Design review of the part shown in the three views and the two pictorial views. Dimensions are in mm from the part's minimum x, y and z. A direction names the side the tool comes from. Give positions to 0.01 mm unless a question says otherwise; leave off trailing zeros. Write each loop counter-clockwise with the first axis right and the second up, starting at its lowest first coordinate (ties: lowest second). Pieces come first, ordered by that corner, then holes.
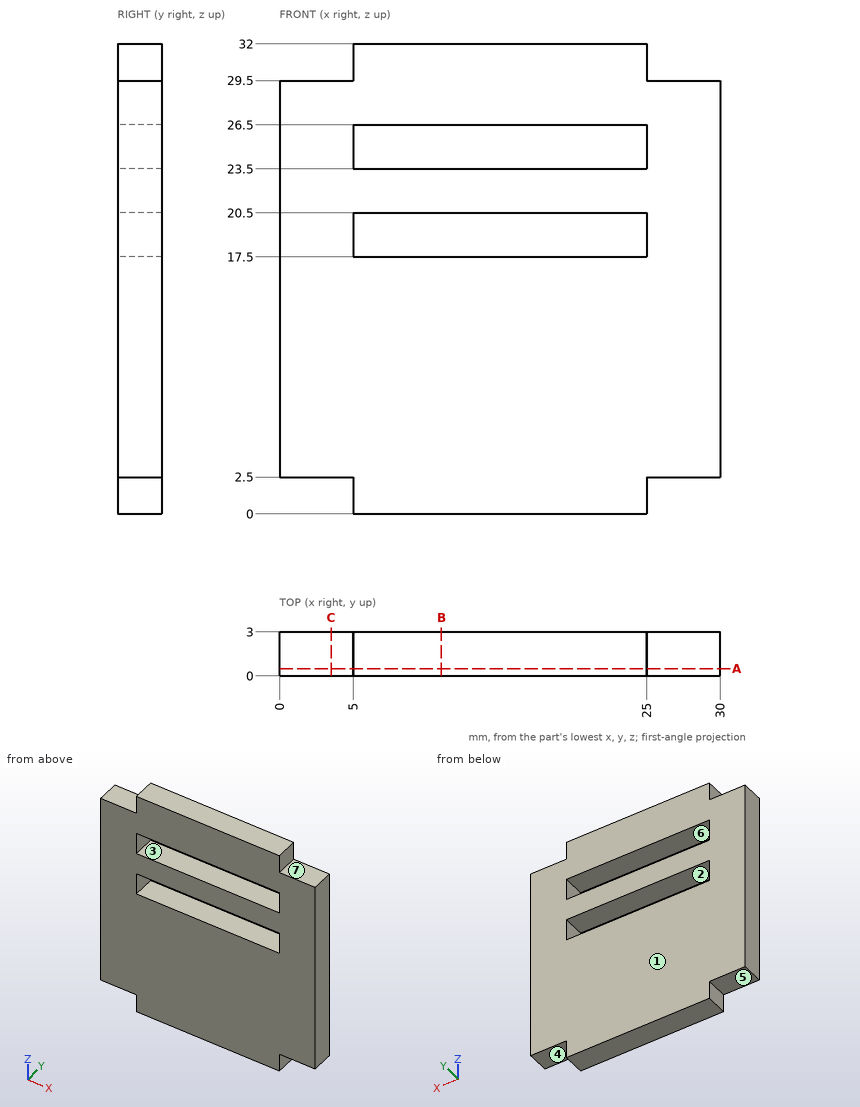
(1) To check wall thickness, follow L1, parallel to Z at x = 20.25, y = 1.6; L2, parallel to X at y = 1, z = 19; L3, parallel to X at y = 0.65, z = 30. State the ranges of each line that lie inside material, in increasing order.
Resolved:
L1: z = 0 to 17.5, 20.5 to 23.5, 26.5 to 32
L2: x = 0 to 5, 25 to 30
L3: x = 5 to 25
(2) Consider section A-A, the plane y = 0.5. Give the boundary of the cut face in (x, z), then the cut area to 3 significant figures.
Resolved:
outline: (0, 2.5) - (5, 2.5) - (5, 0) - (25, 0) - (25, 2.5) - (30, 2.5) - (30, 29.5) - (25, 29.5) - (25, 32) - (5, 32) - (5, 29.5) - (0, 29.5) - close; hole (5, 17.5) - (25, 17.5) - (25, 20.5) - (5, 20.5) - close; hole (5, 23.5) - (25, 23.5) - (25, 26.5) - (5, 26.5) - close
area: 790 mm2
(3) Mouldability with a two-part tool opening along X and no side actions: class the marked faces 1, 2 and 3 as pulls with the +X half, pulls with the -X half, needs draft (parallel to the pull), parting line crosses it, or undercut.
Resolved:
face 1: needs draft
face 2: undercut
face 3: undercut
(4) Consider section B-B, the plane x = 11. Give the boundary of the cut face in (y, z), then the cut area to 3 significant figures.
Resolved:
outline: (0, 0) - (3, 0) - (3, 17.5) - (0, 17.5) - close; (0, 20.5) - (3, 20.5) - (3, 23.5) - (0, 23.5) - close; (0, 26.5) - (3, 26.5) - (3, 32) - (0, 32) - close
area: 78.0 mm2
(5) Consider section C-C, the plane x = 3.5. Give the boundary of the cut face in (y, z), then the cut area to 3 significant figures.
Resolved:
outline: (0, 2.5) - (3, 2.5) - (3, 29.5) - (0, 29.5) - close
area: 81.0 mm2
(6) Clearance check with flat-ended pins moving along their axes: P1, Ø0.8, axis at y = 1.5, z = 30, coming from the +X side; P2, Ø1.5, axis at x = 28, y = 1.5, coming from the -Z side. State where each tip first meets the part, or that it passes through.
Resolved:
P1: stops at x = 25
P2: stops at z = 2.5
(7) Tool access review of the marked faces 4, 5, 6 and 7: name each direction out of +Z, -Z, +X, -X, +Y, -Y from which nothing blocks a thin tool from reaching the whole face with its end or side.
Resolved:
face 4: -Z, +X, +Y, -Y
face 5: -Z, -X, +Y, -Y
face 6: +Y, -Y
face 7: +Z, +X, +Y, -Y
